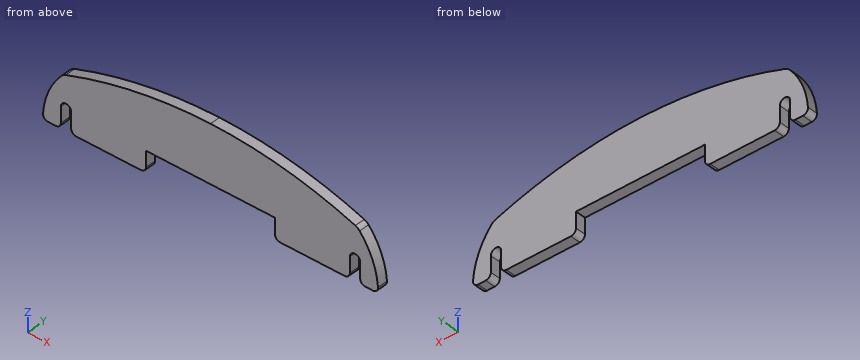
from build123d import *

# Parameters (mm, degrees)
RESSALTO_EXTRUS_O1_DEPTH = 2


with BuildPart() as part:
    # Esboço1 → Ressalto-extrusão1 (new body)
    with BuildSketch(Plane(origin=(0, 0, 0), x_dir=(1, 0, 0), z_dir=(0, 1, 0))):
        with BuildLine():
            Line((-12.5, 0), (12.5, 0))
            Line((12.5, 0), (12.5, 3))
            ThreePointArc((12.5, 3), (12.792893219, 3.707106781), (13.5, 4))
            Line((13.5, 4), (26, 4))
            ThreePointArc((26, 4), (26.707106781, 3.707106781), (27, 3))
            Line((27, 3), (27, 0))
            ThreePointArc((27, 0), (28, -1), (29, 0))
            Line((29, 0), (29, 3))
            ThreePointArc((29, 3), (29.292893219, 3.707106781), (30, 4))
            Line((30, 4), (31.463239539, 4))
            ThreePointArc((31.463239539, 4), (32.195845062, 3.680653471), (32.460540524, 2.926578296))
            ThreePointArc((32.460540524, 2.926578296), (31.37483832, -1.624378023), (28.907100926, -5.599327689))
            ThreePointArc((28.907100926, -5.599327689), (28.523980806, -5.93948611), (28.067011203, -6.171148708))
            ThreePointArc((28.067011203, -6.171148708), (14.239688573, -9.783983548), (0, -11))
            ThreePointArc((0, -11), (-14.239688573, -9.783983548), (-28.067011203, -6.171148708))
            ThreePointArc((-28.067011203, -6.171148708), (-28.523980806, -5.93948611), (-28.907100926, -5.599327689))
            ThreePointArc((-28.907100926, -5.599327689), (-31.37483832, -1.624378023), (-32.460540524, 2.926578296))
            ThreePointArc((-32.460540524, 2.926578296), (-32.195845062, 3.680653471), (-31.463239539, 4))
            Line((-31.463239539, 4), (-30, 4))
            ThreePointArc((-30, 4), (-29.292893219, 3.707106781), (-29, 3))
            Line((-29, 3), (-29, 0))
            ThreePointArc((-29, 0), (-28, -1), (-27, 0))
            Line((-27, 0), (-27, 3))
            ThreePointArc((-27, 3), (-26.707106781, 3.707106781), (-26, 4))
            Line((-26, 4), (-13.5, 4))
            ThreePointArc((-13.5, 4), (-12.792893219, 3.707106781), (-12.5, 3))
            Line((-12.5, 3), (-12.5, 0))
        make_face()
    extrude(amount=RESSALTO_EXTRUS_O1_DEPTH)


solid = part.part
Work out the finished part from the listing and answer in its coordinate system (mm). Coordinates: 2 decimals unless noted, no trailing zeros. Write each loop counter-clockwise with the first axis right and the second up, starting at its lowest first coordinate (ties: lowest second). Pieces come first, ordered by that corner, then holes. Notation, with made-up numbers: M 65,46.5 L 102,46.5 A32 cw 102,74.5 Z; hole C 3.5,6 d8. An arc over 180 degrees is marked long. Answer as CSV lines item,"result". Start each with the question number.
Item 1: Flat-ended cylindrical pins translate along their axes: P1, Ø1, axis at y = 0.5, z = -2, coming from the -X side; P2, Ø0.6, axis at y = 1, z = -1.5, coming from the -X side; P3, Ø1, axis at x = 17, z = 1.5, coming from the -Y side; P4, Ø0.6, axis at y = 1, z = -1, coming from the +X side. Find the tip coordinate at first contact, or state that the pin passes through.
Item 2: Consider L1, parallel to X at y = 0.55, z = 0.75; L2, parallel to X at y = 1.65, z = -1.25; L3, parallel to X at y = 1, z = -0.5. Determine where each line is inside the solid, lowest interval first.
Item 3: Section B-B on z = 8.75 is taken. Write down the section's boundary in (x, y).
Item 4: Section C-C on x = -1.5 is taken. Write down the section's boundary in (y, z).
Item 5: Section A-A on y = 1.7 is taken. Write down the section's boundary in (x, z).
Checks:
1,P1,"stops at x = -32.42"
1,P2,"stops at x = -32.33"
1,P3,"stops at y = 0"
1,P4,"stops at x = 32.25"
2,L1,"x = -31.71 to -28.66, -27.34 to 27.34, 28.66 to 31.71"
2,L2,"x = -32.24 to -29, -27 to -12.5, 12.5 to 27, 29 to 32.24"
2,L3,"x = -32.07 to -29, -27 to -12.5, 12.5 to 27, 29 to 32.07"
3,outline,"M -19.31,0 L 19.31,0 L 19.31,2 L -19.31,2 Z"
4,outline,"M 0,0 L 2,0 L 2,10.99 L 0,10.99 Z"
5,outline,"M -32.46,-2.93 A1 ccw -31.46,-4 L -30,-4 A1 ccw -29,-3 L -29,0 A1 cw -27,0 L -27,-3 A1 ccw -26,-4 L -13.5,-4 A1 ccw -12.5,-3 L -12.5,0 L 12.5,0 L 12.5,-3 A1 ccw 13.5,-4 L 26,-4 A1 ccw 27,-3 L 27,0 A1 cw 29,0 L 29,-3 A1 ccw 30,-4 L 31.46,-4 A1 ccw 32.46,-2.93 A14.62 ccw 28.91,5.6 A2 ccw 28.07,6.17 A83.98 ccw -28.07,6.17 A2 ccw -28.91,5.6 A14.62 ccw Z"
